Input: part model. Units: mm. Frame: model coordinates. Face numbers are marked on the shaded views. A direction names the side the tool comes from. Round coordinates to 2 decimals unless told otherwise and drop trailing zeros. Loops run counter-clockwise (first coordinate to the right, second up) from the corner with the lowest first, then second, coordinate; pieces in that order, holes last. Notation, with made-up numbers: (-21.75, 77.5) -> (-11.75, 77.5) arc R9 ccw to (-11.75, 94.5) -> close; hole circle Ø1 at (43.5, -23.5). An arc over 180 degrees is marked (long way). Answer in a Markdown table with one row per item. Add a question column.
Q1. Section C-C, the plane z = 0.55. Output: boundary loops of the cut face in (x, y).
Q2. Section A-A, the plane y = 0. Output: boundary loops of the cut face in (x, z), and give its area (3 significant figures).
Q3. Reachability of the marked faces 1 and 2 from +Z, -Z, +X, -X, +Y, -Y: full face, straight path, thin tool, end or side. Return the list, or none.
Q4. Section D-D, the plane y = -7. Output: boundary loops of the cut face in (x, z).
Q5. Pin query (flat end, axial travel): pin 1 (2 mm diameter, centred on y = -6.5, z = 4, fed in from +X); pin 2 (4.5 mm diameter, centred on x = 0, y = 0, fed in from +Z). Return the tip coordinate at first contact, or that it passes through.
Q6. Mould query, pull axis Y, two halves, no side actions, for the marked faces 3, 4, 5 and 6. Classes: pulls with the +Y half, pulls with the -Y half, needs draft (parallel to the pull), parting line crosses it, or undercut.
Q7. Ray query, L1, parallel to X at y = 7, z = 0.6; L2, parallel to Y at x = 6.25, z = 2.45; L3, parallel to Z at x = -6.5, y = -1.5. Return the intervals inside material, ascending. Write a range as from..to.
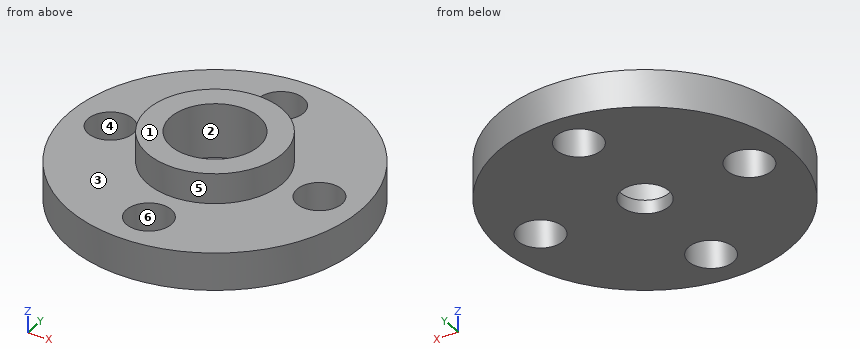
```python
from build123d import *

# Parameters (mm, degrees)
SKETCH_1_R               = 9.75
EXTRUDE_1_DEPTH          = 2.5
SKETCH_2_R               = 4.5
EXTRUDE_2_DEPTH          = 2
SKETCH_3_R               = 2.95
CUT_EXTRUDE_1_DEPTH      = 3.6
SKETCH_4_R               = 1.6
CUT_EXTRUDE_2_DEPTH      = 3.6
SKETCH_5_R               = 1.5
CUT_EXTRUDE_3_DEPTH      = 15.013386457
PATTERN_CIRCULAR_1_COUNT = 4


with BuildPart() as part:
    # 草图1 → 凸台-拉伸1 (new body)
    with BuildSketch(Plane.XY):
        Circle(SKETCH_1_R)
    extrude(amount=EXTRUDE_1_DEPTH)

    # 草图2 → 凸台-拉伸2 (add)
    with BuildSketch(Plane.XY.offset(2.5)):
        Circle(SKETCH_2_R)
    extrude(amount=EXTRUDE_2_DEPTH)

    # 草图3 → 切除-拉伸1 (cut)
    with BuildSketch(Plane.XY.offset(4.5)):
        Circle(SKETCH_3_R)
    extrude(amount=-CUT_EXTRUDE_1_DEPTH, mode=Mode.SUBTRACT)

    # 草图4 → 切除-拉伸2 (cut)
    with BuildSketch(Plane(origin=(0, 0, 0), x_dir=(-1, 0, 0), z_dir=(0, 0, -1))):
        Circle(SKETCH_4_R)
    extrude(amount=-CUT_EXTRUDE_2_DEPTH, mode=Mode.SUBTRACT)

    # 草图5 → 切除-拉伸3 (cut, through all)
    with BuildSketch(Plane.XY.offset(2.5)):
        with Locations((-7, 0)):
            Circle(SKETCH_5_R)
    cut_extrude_3 = extrude(amount=-CUT_EXTRUDE_3_DEPTH, mode=Mode.SUBTRACT)

    # 阵列(圆周)1: 切除-拉伸3 ×4 about axis
    pattern_circular_1_axis = Axis((0, 0, 0), (0, 0, 1))
    for i in range(1, PATTERN_CIRCULAR_1_COUNT):
        add(cut_extrude_3.rotate(pattern_circular_1_axis, i * 360 / PATTERN_CIRCULAR_1_COUNT), mode=Mode.SUBTRACT)


solid = part.part
```
Answer block:
| question | item | result |
|---|---|---|
| 1 | outline | circle Ø19.5 at (0, 0); hole circle Ø3 at (-7, 0); hole circle Ø3.2 at (0, 0); hole circle Ø3 at (0, -7); hole circle Ø3 at (0, 7); hole circle Ø3 at (7, 0) |
| 2 | outline | (-9.75, 0) -> (-8.5, 0) -> (-8.5, 2.5) -> (-9.75, 2.5) -> close; (-5.5, 0) -> (-1.6, 0) -> (-1.6, 0.9) -> (-2.95, 0.9) -> (-2.95, 4.5) -> (-4.5, 4.5) -> (-4.5, 2.5) -> (-5.5, 2.5) -> close; (1.6, 0) -> (5.5, 0) -> (5.5, 2.5) -> (4.5, 2.5) -> (4.5, 4.5) -> (2.95, 4.5) -> (2.95, 0.9) -> (1.6, 0.9) -> close; (8.5, 0) -> (9.75, 0) -> (9.75, 2.5) -> (8.5, 2.5) -> close |
| 2 | area | 27.6 mm^2 |
| 3 | face 1 | +Z, +X, -X, +Y, -Y |
| 3 | face 2 | +Z |
| 4 | outline | (-6.79, 0) -> (-1.5, 0) -> (-1.5, 2.5) -> (-6.79, 2.5) -> close; (1.5, 0) -> (6.79, 0) -> (6.79, 2.5) -> (1.5, 2.5) -> close |
| 5 | pin 1 | through |
| 5 | pin 2 | z = 0.9 |
| 6 | face 3 | needs draft |
| 6 | face 4 | undercut |
| 6 | face 5 | parting line crosses it |
| 6 | face 6 | undercut |
| 7 | L1 | -6.79..-1.5, 1.5..6.79 |
| 7 | L2 | -7.48..-1.3, 1.3..7.48 |
| 7 | L3 | 0..2.5 |
